```python
from build123d import *

# Parameters (mm, degrees)
SKETCH1_W                = 30
SKETCH1_H                = 30
SKETCH1_W_2              = 7
SKETCH1_H_2              = 26
BOSS_EXTRUDE3_DEPTH      = 110
BOSS_EXTRUDE3_DEPTH_BACK = 80
SKETCH6_R                = 12.7
CUT_EXTRUDE5_DEPTH       = 23
SKETCH8_R                = 3.6
SKETCH8_R_2              = 1.7
CUT_EXTRUDE6_DEPTH       = 17
SKETCH9_W                = 12
SKETCH9_H                = 26
CUT_EXTRUDE7_DEPTH       = 155
M3_CLEARANCE_HOLE1_D     = 3.6


with BuildPart() as part:
    # Sketch1 → Boss-Extrude3 (new body, two sides)
    with BuildSketch(Plane(origin=(0, 0, 0), x_dir=(0, 0, -1), z_dir=(1, 0, 0))) as boss_extrude3_sk:
        Rectangle(SKETCH1_W, SKETCH1_H)
        with Locations((-9.5, 0)):
            Rectangle(SKETCH1_W_2, SKETCH1_H_2, mode=Mode.SUBTRACT)
        with Locations((9.5, 0)):
            Rectangle(SKETCH1_W_2, SKETCH1_H_2, mode=Mode.SUBTRACT)
    extrude(amount=BOSS_EXTRUDE3_DEPTH)
    extrude(boss_extrude3_sk.sketch, amount=-BOSS_EXTRUDE3_DEPTH_BACK)

    # Sketch6 → Cut-Extrude5 (cut)
    with BuildSketch(Plane(origin=(0, 0, -15), x_dir=(-1, 0, 0), z_dir=(0, 0, -1))):
        with Locations((-95, 0)):
            Circle(SKETCH6_R)
    extrude(amount=-CUT_EXTRUDE5_DEPTH, mode=Mode.SUBTRACT)

    # Sketch8 → Cut-Extrude6 (cut)
    with BuildSketch(Plane.XY.offset(15)):
        with Locations((95, 0)):
            Circle(SKETCH8_R)
        with Locations((95, 8.5)):
            Circle(SKETCH8_R_2)
        with Locations((95, -8.5)):
            Circle(SKETCH8_R_2)
    extrude(amount=-CUT_EXTRUDE6_DEPTH, mode=Mode.SUBTRACT)

    # Sketch9 → Cut-Extrude7 (cut)
    with BuildSketch(Plane.ZY.offset(80)):
        Rectangle(SKETCH9_W, SKETCH9_H)
    extrude(amount=-CUT_EXTRUDE7_DEPTH, mode=Mode.SUBTRACT)

    # M3 Clearance Hole1 (through all)
    with Locations(Plane.XY.offset(15)):
        with Locations((-75, 10), (-75, -10), (-55, -10), (-55, 10)):
            Hole(M3_CLEARANCE_HOLE1_D / 2)


solid = part.part
```
Could you check a few things on this model? Use its own coordinates, in mm. A direction names the side the tool comes from. Coordinates: 2 decimals unless noted, no trailing zeros. Order: outer loops, then holes, each group sorted by start corner. A loop starts at its lowest first (then second) coordinate and runs counter-clockwise, first axis right, second up. Notation, with made-up numbers: M 53,-29.75 L 75,-29.75 A15 ccw 75,-22.75 Z; hole C -17.75,-28 d10. An arc over 180 degrees is marked long. Use one line per item in the form item = value. Start each with the question number.
1. Suppose I cut it at A-A on x = -35. Write out the boundary of the cut face in (y, z), then the cut area to 3 significant figures.
2. Suppose I cut it at B-B on x = 95. Count the separate pieces of the cut face and the enclosed holes in it, then the cut area to 3 significant figures.
3. We'd pull the mould along X, two halves only. Please class faces 6 (the flat face through (16, 0, -15)), 7 (the cylindrical face through (-73.572, 8.905, -14.014)), 8 (the flat face through (75, 0, 0)), 9 (the cylindrical face through (107.688, 0.558, -0.084)): +X half, -X half, draft (parallel to the pull), parting line (faces both ways), or undercut.
4. Please list where these lines run through material, in increasing order: line 1 (Y direction, x = 95, z = 13.85); line 2 (Y direction, x = -75, z = -13.45); line 3 (Y direction, x = 59, z = 8).
5. On a 3-axis mill with a long thin cutter (end or side, diameter ignored), from which of +Z, -Z, +X, -X, +Y, -Y can I reach the whole of each face in a straight line? I mean faces 1 (the cylindrical face through (-55.831, -11.597, 13.986)), 2 (the flat face through (16, 13, 0)), 3 (the flat face through (81, 0, -6)), 4 (the flat face through (110, 0, 0)), 5 (the cylindrical face through (107.688, 0.558, -14.014)). Say none if no direction works.
6. For pin 1 (8 mm diameter, centred on x = 94, y = -0.5, fed in from -Z), with a flat end and sliding along its axis, tell me the tip position at first contact or that it passes through.
7. Suppose I cut it at C-C on x = -75. Write out the boundary of the cut face in (y, z), then the cut area to 3 significant figures.
Geometry says:
q1.outline = M -15,-15 L 15,-15 L 15,15 L -15,15 Z; hole M -13,-13 L 13,-13 L 13,13 L -13,13 Z
q1.area = 224 mm^2
q2.separate_pieces = 4
q2.enclosed_holes = 0
q2.area = 152 mm^2
q3.face_6 = draft
q3.face_7 = undercut
q3.face_8 = -X half
q3.face_9 = undercut
q4.line_1 = -15 to -10.2, -6.8 to -3.6, 3.6 to 6.8, 10.2 to 15
q4.line_2 = -15 to -11.8, -8.2 to 8.2, 11.8 to 15
q4.line_3 = -15 to -13, 13 to 15
q5.face_1 = +Z, -Z
q5.face_2 = -X
q5.face_3 = +X, -X
q5.face_4 = +Z, -Z, +X, +Y, -Y
q5.face_5 = -Z
q6.pin_1 = 13
q7.outline = M -15,-15 L -11.8,-15 L -11.8,-13 L -13,-13 L -13,13 L -11.8,13 L -11.8,15 L -15,15 Z; M -8.2,-15 L 8.2,-15 L 8.2,-13 L -8.2,-13 Z; M -8.2,13 L 8.2,13 L 8.2,15 L -8.2,15 Z; M 11.8,-15 L 15,-15 L 15,15 L 11.8,15 L 11.8,13 L 13,13 L 13,-13 L 11.8,-13 Z
q7.area = 195 mm^2
